from build123d import *

# Parameters (mm, degrees)
BOSS_EXTRUDE1_DEPTH = 60
CUT_EXTRUDE1_REACH  = 104.837
SKETCH2_R           = 6
CUT_EXTRUDE2_REACH  = 105.923
SKETCH3_R           = 3
SKETCH3_W           = 28
SKETCH3_H           = 10
SKETCH4_R           = 3
SKETCH4_W           = 28
SKETCH4_H           = 10
CUT_EXTRUDE3_DEPTH  = 60


with BuildPart() as part:
    # Sketch1 → Boss-Extrude1 (new body)
    with BuildSketch(Plane(origin=(0, 0, 0), x_dir=(0, 0, -1), z_dir=(1, 0, 0))):
        with BuildLine():
            Line((-55, 60), (-55, 55))
            Line((-55, 55), (-34.537682266, 55))
            ThreePointArc((-34.537682266, 55), (-32.471600854, 54.55316457), (-30.774798792, 53.292523039))
            Line((-30.774798792, 53.292523039), (-1.237116526, 19.535171878))
            ThreePointArc((-1.237116526, 19.535171878), (-0.31948628, 18.001282205), (0, 16.242648839))
            Line((0, 16.242648839), (0, 0))
            Line((0, 0), (5, 0))
            Line((5, 0), (5, 20))
            Line((5, 20), (-30, 60))
            Line((-30, 60), (-55, 60))
        make_face()
    extrude(amount=BOSS_EXTRUDE1_DEPTH)

    # Sketch2 → Cut-Extrude1 (cut, up to next)
    with BuildSketch(Plane(origin=(0, 11.150442478, -12.743362832), x_dir=(-1, 0, 0), z_dir=(0, 0.6585046078685178, -0.752576694706878)), mode=Mode.PRIVATE) as cut_extrude1_sk1:
        with Locations(Location((-40, 48.334739918, 0), (0, 0, 90))):
            Circle(SKETCH2_R)
    cut_extrude1_tool1 = extrude(cut_extrude1_sk1.sketch, amount=-CUT_EXTRUDE1_REACH, mode=Mode.PRIVATE) & part.part
    # Sketch2 → Cut-Extrude1 (cut, up to next)
    with BuildSketch(Plane(origin=(0, 11.150442478, -12.743362832), x_dir=(-1, 0, 0), z_dir=(0, 0.6585046078685178, -0.752576694706878)), mode=Mode.PRIVATE) as cut_extrude1_sk2:
        with Locations(Location((-40, 28.334739918, 0), (0, 0, 90))):
            Circle(SKETCH2_R)
    cut_extrude1_tool2 = extrude(cut_extrude1_sk2.sketch, amount=-CUT_EXTRUDE1_REACH, mode=Mode.PRIVATE) & part.part
    # Sketch2 → Cut-Extrude1 (cut, up to next)
    with BuildSketch(Plane(origin=(0, 11.150442478, -12.743362832), x_dir=(-1, 0, 0), z_dir=(0, 0.6585046078685178, -0.752576694706878)), mode=Mode.PRIVATE) as cut_extrude1_sk3:
        with Locations(Location((-20, 48.334739918, 0), (0, 0, 90))):
            Circle(SKETCH2_R)
    cut_extrude1_tool3 = extrude(cut_extrude1_sk3.sketch, amount=-CUT_EXTRUDE1_REACH, mode=Mode.PRIVATE) & part.part
    # Sketch2 → Cut-Extrude1 (cut, up to next)
    with BuildSketch(Plane(origin=(0, 11.150442478, -12.743362832), x_dir=(-1, 0, 0), z_dir=(0, 0.6585046078685178, -0.752576694706878)), mode=Mode.PRIVATE) as cut_extrude1_sk4:
        with Locations(Location((-20, 28.334739918, 0), (0, 0, 90))):
            Circle(SKETCH2_R)
    cut_extrude1_tool4 = extrude(cut_extrude1_sk4.sketch, amount=-CUT_EXTRUDE1_REACH, mode=Mode.PRIVATE) & part.part
    add(cut_extrude1_tool1.solids().sort_by_distance((40, 47.526041, 19.085286))[0], mode=Mode.SUBTRACT)
    add(cut_extrude1_tool2.solids().sort_by_distance((40, 32.474507, 5.915194))[0], mode=Mode.SUBTRACT)
    add(cut_extrude1_tool3.solids().sort_by_distance((20, 47.526041, 19.085286))[0], mode=Mode.SUBTRACT)
    add(cut_extrude1_tool4.solids().sort_by_distance((20, 32.474507, 5.915194))[0], mode=Mode.SUBTRACT)

    # Sketch3 → Cut-Extrude2 (cut, up to next)
    with BuildSketch(Plane(origin=(0, 0, -5), x_dir=(-1, 0, 0), z_dir=(0, 0, -1)), mode=Mode.PRIVATE) as cut_extrude2_sk1:
        with Locations((-52, 5)):
            Circle(SKETCH3_R)
    cut_extrude2_tool1 = extrude(cut_extrude2_sk1.sketch, amount=-CUT_EXTRUDE2_REACH, mode=Mode.PRIVATE) & part.part
    # Sketch3 → Cut-Extrude2 (cut, up to next)
    with BuildSketch(Plane(origin=(0, 0, -5), x_dir=(-1, 0, 0), z_dir=(0, 0, -1)), mode=Mode.PRIVATE) as cut_extrude2_sk2:
        with Locations((-10, 5)):
            Circle(SKETCH3_R)
    cut_extrude2_tool2 = extrude(cut_extrude2_sk2.sketch, amount=-CUT_EXTRUDE2_REACH, mode=Mode.PRIVATE) & part.part
    # Sketch3 → Cut-Extrude2 (cut, up to next)
    with BuildSketch(Plane(origin=(0, 0, -5), x_dir=(-1, 0, 0), z_dir=(0, 0, -1)), mode=Mode.PRIVATE) as cut_extrude2_sk3:
        with Locations((-30, 5)):
            Rectangle(SKETCH3_W, SKETCH3_H)
    cut_extrude2_tool3 = extrude(cut_extrude2_sk3.sketch, amount=-CUT_EXTRUDE2_REACH, mode=Mode.PRIVATE) & part.part
    add(cut_extrude2_tool1.solids().sort_by_distance((52, 5, -5))[0], mode=Mode.SUBTRACT)
    add(cut_extrude2_tool2.solids().sort_by_distance((10, 5, -5))[0], mode=Mode.SUBTRACT)
    add(cut_extrude2_tool3.solids().sort_by_distance((30, 5, -5))[0], mode=Mode.SUBTRACT)

    # Sketch4 → Cut-Extrude3 (cut)
    with BuildSketch(Plane(origin=(0, 60, 0), x_dir=(1, 0, 0), z_dir=(0, 1, 0))):
        with Locations(Location((8, -50, 0), (0, 0, 270))):
            Circle(SKETCH4_R)
        with Locations(Location((52, -50, 0), (0, 0, 270))):
            Circle(SKETCH4_R)
        with Locations((30, -50)):
            Rectangle(SKETCH4_W, SKETCH4_H)
    extrude(amount=-CUT_EXTRUDE3_DEPTH, mode=Mode.SUBTRACT)


solid = part.part
Build history of the part. All positions in model axes, mm. A direction names the side the tool comes from. Round coordinates to 2 decimals unless told otherwise and drop trailing zeros. Loops run counter-clockwise (first coordinate to the right, second up) from the corner with the lowest first, then second, coordinate; pieces in that order, holes last. Notation, with made-up numbers: (16, 32) -> (31, 32) arc R25 cw to (31, 54) -> close; hole circle Ø9 at (20.5, -6). An arc over 180 degrees is marked (long way). One line per item, written item: value. Start each with the question number.
Q1. Cut at C-C on y = 6. List the corners of the cut face in (x, z), plus the area to 3 significant figures.
Q2. Cut at B-B on x = 52. List the corners of the cut face in (y, z), plus the area to 3 significant figures.
Q3. Cut at D-D on x = 25. List the corners of the cut face in (y, z).
Q4. 3-axis set-ups, long thin cutter, end or side, ignore diameter. For faces 1 (the face through (30, 55, 43)), 2 (the face through (34.143, 29.872, 6.914)), 3 (the face through (16, 5, -3)), 4 (the face through (16, 58, 50)): which of +Z, -Z, +X, -X, +Y, -Y reach the whole face in a straight line?
Q5. Drop flat-ended pins along their axis: pin 1 Ø1 at (x, z) = (48.5, 4) entering from +Y; pin 2 Ø6 at (x, z) = (17.5, 46) entering from -Y; pin 3 Ø5 at (x, z) = (6.5, 33.5) entering from -Y; pin 4 Ø5.5 at (x, z) = (52, 50) entering from +Y. Give the stop position or say it passes through.
Q6. Two-plate mould, pull along X, no slides. Class faces 5 (the face through (21.8, 50.21, 24.71)), 6 (the face through (60, 37, 16)), 7 (the face through (29.58, 36.65, 16.21)): released by +X, released by -X, zero draft, split by the parting line, or undercut.
Q7. Probe line 1 along X through (y, z) = (34.5, 12); line 2 along Y through (x, z) = (10, -2.75); line 3 along Y through (x, z) = (10, -1.55). List the from-to ranges inside material, lowest first.
Q8. Cut at A-A on z = 50. List the corners of the cut face in (x, y).
Computed:
1. outline: (0, -5) -> (7.17, -5) -> (7.17, 0) -> (0, 0) -> close; (12.83, -5) -> (16, -5) -> (16, 0) -> (12.83, 0) -> close; (44, -5) -> (49.17, -5) -> (49.17, 0) -> (44, 0) -> close; (54.83, -5) -> (60, -5) -> (60, 0) -> (54.83, 0) -> close
1. area: 103 mm²
2. outline: (0, -5) -> (2, -5) -> (2, 0) -> (0, 0) -> close; (8, -5) -> (20, -5) -> (60, 30) -> (60, 47) -> (55, 47) -> (55, 34.54) arc R5 cw to (53.29, 30.77) -> (19.54, 1.24) arc R5 cw to (16.24, 0) -> (8, 0) -> close; (55, 53) -> (60, 53) -> (60, 55) -> (55, 55) -> close
2. area: 411 mm²
3. outline: (10, -5) -> (20, -5) -> (29.98, 3.73) -> (26.69, 7.49) -> (19.54, 1.24) arc R5 cw to (16.24, 0) -> (10, 0) -> close; (31.68, 11.86) -> (34.97, 8.1) -> (45.03, 16.9) -> (41.74, 20.66) -> close; (46.73, 25.03) -> (50.02, 21.27) -> (60, 30) -> (60, 45) -> (55, 45) -> (55, 34.54) arc R5 cw to (53.29, 30.77) -> close
4. face 1: +Z, +X, -X, -Y
4. face 2: none
4. face 3: +Z, -Z, -Y
4. face 4: +Z, +Y, -Y
5. pin 1: y = 30.86
5. pin 2: y = 55
5. pin 3: y = 53.53
5. pin 4: through
6. face 5: undercut
6. face 6: released by +X
6. face 7: zero draft
7. line 1: 0 to 17.67, 22.33 to 37.67, 42.33 to 60
7. line 2: 0 to 2, 8 to 22.57
7. line 3: 0 to 2, 8 to 23.94
8. outline: (0, 55) -> (5, 55) -> (5, 60) -> (0, 60) -> close; (11, 55) -> (16, 55) -> (16, 60) -> (11, 60) -> close; (44, 55) -> (49, 55) -> (49, 60) -> (44, 60) -> close; (55, 55) -> (60, 55) -> (60, 60) -> (55, 60) -> close
